Could you check a few things on this model? Use its own coordinates, in mm. Coordinates: 2 decimals unless noted, no trailing zeros. Write each loop counter-clockwise with the first axis right and the second up, starting at its lowest first coordinate (ties: lowest second). Pieces come first, ordered by that corner, then holes. Notation, with made-up numbers: M 75.25,32.25 L 124.25,32.25 A21 cw 124.25,55.25 Z; hole C 71.25,47.25 d10. An arc over 180 degrees is marked long. Write item = value, one per line.
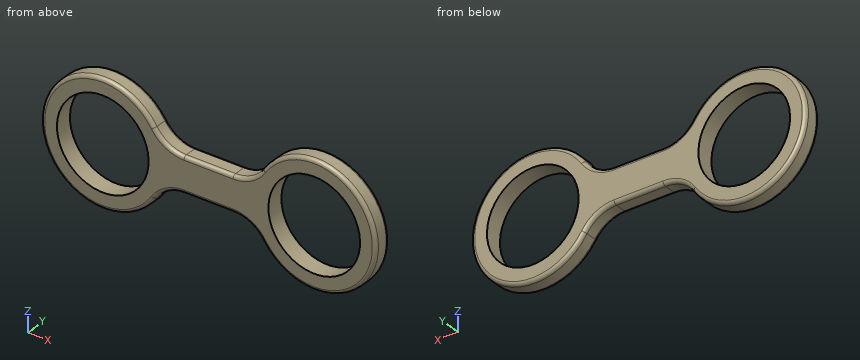
```python
from build123d import *

# Parameters (mm, degrees)
SKETCH1_R           = 13
BOSS_EXTRUDE1_DEPTH = 5
FILLET1_R           = 10
FILLET2_R           = 1


with BuildPart() as part:
    # Sketch1 → Boss-Extrude1 (new body)
    with BuildSketch(Plane(origin=(0, 0, 0), x_dir=(1, 0, 0), z_dir=(0, 1, 0))):
        with BuildLine():
            Line((16.770509831, 5), (43.229490169, 5))
            ThreePointArc((43.229490169, 5), (77.5, 0), (43.229490169, -5))
            Line((43.229490169, -5), (16.770509831, -5))
            ThreePointArc((16.770509831, -5), (-17.5, 0), (16.770509831, 5))
        make_face()
        with Locations(Location((0, 0, 0), (0, 0, 270))):
            Circle(SKETCH1_R, mode=Mode.SUBTRACT)
        with Locations(Location((60, 0, 0), (0, 0, 270))):
            Circle(SKETCH1_R, mode=Mode.SUBTRACT)
    extrude(amount=BOSS_EXTRUDE1_DEPTH)

    # Fillet1
    fillet1_edges = [part.edges().sort_by_distance(p)[0] for p in [
        (16.770509831, 2.5, -5),
        (43.229490169, 2.5, -5),
        (43.229490169, 2.5, 5),
        (16.770509831, 2.5, 5),
    ]]
    fillet(fillet1_edges, radius=FILLET1_R)

    # Fillet2
    fillet2_edges = [part.edges().sort_by_distance(p)[0] for p in [
        (77.5, 0, 0),
        (77.5, 5, 0),
        (30, 0, 5),
        (30, 5, 5),
        (-17.5, 0, 0),
        (-17.5, 5, 0),
        (30, 0, -5),
        (30, 5, -5),
        (41.718451803, 0, 6.20950927),
        (41.718451803, 5, 6.20950927),
        (18.281548197, 0, 6.20950927),
        (18.281548197, 5, 6.20950927),
        (41.718451803, 0, -6.20950927),
        (41.718451803, 5, -6.20950927),
        (18.281548197, 0, -6.20950927),
        (18.281548197, 5, -6.20950927),
    ]]
    fillet(fillet2_edges, radius=FILLET2_R)


solid = part.part
```
Item 1: Imagine slicing it at B-B (x = 34). Write out the boundary of the cut face in (y, z).
Numbers:
outline = M 0,-4 A1 ccw 1,-5 L 4,-5 A1 ccw 5,-4 L 5,4 A1 ccw 4,5 L 1,5 A1 ccw 0,4 Z
Item 2: I'm going to push a flat-ended pin straight in: P1, Ø1.5, axis at x = 28.5, y = 2.5, coming from the -Z side. Where does the tip first touch, or does it pass through?
Numbers:
P1 = -5
Item 3: Imagine slicing it at A-A (z = 0). Write out the boundary of the cut face in (x, y), and give its area (3 significant figures).
Numbers:
outline = M -17.5,1 A1 ccw -16.5,0 L -13,0 L -13,5 L -16.5,5 A1 ccw -17.5,4 Z; M 13,0 L 47,0 L 47,5 L 13,5 Z; M 73,0 L 76.5,0 A1 ccw 77.5,1 L 77.5,4 A1 ccw 76.5,5 L 73,5 Z
area = 214 mm²
Item 4: If I drill on line 1 along X through (y, z) = (2.9, 0); line 2 along X through (y, z) = (2.9, -8); line 3 along X through (y, z) = (4.7, -6), over which ranges is the centre line in solid material (lowest first)?
Numbers:
line_1 = -17.5 to -13, 13 to 47, 73 to 77.5
line_2 = -15.56 to -10.25, 10.25 to 15.91, 44.09 to 49.75, 70.25 to 75.56
line_3 = -16.13 to -11.53, 11.53 to 18.07, 41.93 to 48.47, 71.53 to 76.13
Item 5: Imagine slicing it at C-C (z = -8). State how many separate pieces and enclosed holes the cut face has, and give its area (3 significant figures).
Numbers:
separate_pieces = 4
enclosed_holes = 0
area = 108 mm²
